Geometry check sheet. Reference: the model listing, model coordinates, mm. A direction names the side the tool comes from. Coordinates: 2 decimals unless noted, no trailing zeros. Loops run counter-clockwise (first coordinate to the right, second up) from the corner with the lowest first, then second, coordinate; pieces in that order, holes last.
Autodesk Fusion 360 part; units mm, degrees
sketch "Sketch1" plane through (0, 0, 0) normal (0, 0, 1) x (1, 0, 0)
  circle A0 centre (0, 0) radius 5.25
  circle A1 centre (0, 0) radius 6.5
  dimension "d1" = 10.5
  dimension "d2" = 1.25
sketch "Sketch2" plane through (0, 0, 0) normal (0, 0, 1) x (1, 0, 0)
  arc A0 (3.25, -8.25) -> (8.25, -3.25) centre (3.25, -3.25) ccw
  line L0 (3.25, 7.05) -> (-3.25, 7.05)
  line L1 (-8.25, 8.25) -> (8.25, -8.25) construction
  line L2 (8.25, -3.25) -> (8.25, 3.25)
  line L3 (7.05, -3.25) -> (7.05, 3.25)
  circle A1 centre (0, 0) radius 5.5
  arc A2 (-3.25, 8.25) -> (-8.25, 3.25) centre (-3.25, 3.25) ccw
  line L4 (8.25, 8.25) -> (-8.25, -8.25) construction
  line L5 (-8.25, 3.25) -> (-8.25, -3.25)
  arc A3 (-7.05, -3.25) -> (-3.25, -7.05) centre (-3.25, -3.25) ccw
  line L6 (3.25, 9.25) -> (-3.25, 9.25)
  arc A4 (-8.25, -3.25) -> (-3.25, -8.25) centre (-3.25, -3.25) ccw
  line L7 (-3.25, -7.05) -> (3.25, -7.05)
  arc A5 (8.25, 3.25) -> (3.25, 8.25) centre (3.25, 3.25) ccw
  arc A6 (3.25, -9.25) -> (9.25, -3.25) centre (3.25, -3.25) ccw
  line L8 (3.25, 8.25) -> (-3.25, 8.25)
  line L9 (9.25, -3.25) -> (9.25, 3.25)
  arc A7 (3.25, -7.05) -> (7.05, -3.25) centre (3.25, -3.25) ccw
  arc A8 (-3.25, 7.05) -> (-7.05, 3.25) centre (-3.25, 3.25) ccw
  arc A9 (-9.25, -3.25) -> (-3.25, -9.25) centre (-3.25, -3.25) ccw
  circle A10 centre (0, 0) radius 4.5
  line L10 (-3.25, -9.25) -> (3.25, -9.25)
  arc A11 (7.05, 3.25) -> (3.25, 7.05) centre (3.25, 3.25) ccw
  line L11 (-9.25, 3.25) -> (-9.25, -3.25)
  arc A12 (9.25, 3.25) -> (3.25, 9.25) centre (3.25, 3.25) ccw
  line L12 (-3.25, -8.25) -> (3.25, -8.25)
  arc A13 (-3.25, 9.25) -> (-9.25, 3.25) centre (-3.25, 3.25) ccw
  line L13 (-7.05, 3.25) -> (-7.05, -3.25)
  dimension "d3" = 1
  dimension "d4" = 1.2
  dimension "d5" = 1
  dimension "d6" = 16.5
  dimension "d7" = 16.5
  dimension "d8" = 5
  dimension "d9" = 11
extrude "Extrude1" add sketch "Sketch2" along normal blind 5 contours A0 L2 A2 L5 A4 A5 L8 L12 | A1 makes body 1 at (7.45, 1.0833, 0) makes body 2 at (5.4932, -0.2742, 3.3333)
extrude "Extrude2" add sketch "Sketch2" against normal blind 1 from surface at 5 contours A0 L2 A2 L5 A4 A5 L8 L12 | L0 L3 A3 L7 A7 A8 A11 L13 | A1 | A10 bodies 1 2
extrude "Extrude3" add sketch "Sketch1" along normal blind 13 from surface at 5 bodies 1
ref_plane "WorkPlane1" through (0, -6.5, 9.9379) normal (0, -1, 0) x (-1, 0, 0)
sketch "Sketch3" plane through (0, -6.5, 0) normal (0, -1, 0) x (-1, 0, 0)
  line L0 (0, 0) -> (0, -19) construction
  line L1 (0, 0) -> (0, -5) construction
  line L2 (0, -5) -> (0, -19) construction
  circle A0 centre (0, -12) radius 1.75
  dimension "d19" = 19
  dimension "d20" = 5
  dimension "d21" = 3.5
extrude "Extrude4" cut sketch "Sketch3" against normal blind 4 bodies 1
chamfer "Chamfer1" distance 1 angle 45 1 edges at (-6.0601, 2.3505, 5) on bodies 1
chamfer "Chamfer2" distance 1 angle 45 8 edges at (5.937, -5.937, 4) (7.05, 0, 4) (5.937, 5.937, 4) (0, 7.05, 4) (-5.937, 5.937, 4) (-7.05, 0, 4) (-5.937, -5.937, 4) (0, -7.05, 4) on bodies 1
1) Section check C-C on y = 0. Record the cut outline in (x, z).
Data:
outline: (-8.25, 0) - (-7.05, 0) - (-7.05, 3) - (-6.05, 4) - (-5.5, 4) - (-5.5, 0) - (-4.5, 0) - (-4.5, 4) - (4.5, 4) - (4.5, 0) - (5.5, 0) - (5.5, 4) - (6.05, 4) - (7.05, 3) - (7.05, 0) - (8.25, 0) - (8.25, 5) - (7.5, 5) - (6.5, 6) - (6.5, 18) - (5.25, 18) - (5.25, 5) - (-5.25, 5) - (-5.25, 18) - (-6.5, 18) - (-6.5, 6) - (-7.5, 5) - (-8.25, 5) - close
2) Section check A-A on z = 3.75. Record the cut outline in (x, y).
Data:
outline: (-8.25, -3.25) arc R5 ccw to (-3.25, -8.25) - (3.25, -8.25) arc R5 ccw to (8.25, -3.25) - (8.25, 3.25) arc R5 ccw to (3.25, 8.25) - (-3.25, 8.25) arc R5 ccw to (-8.25, 3.25) - close; circle Ø11 at (0, 0); hole (-6.3, -3.25) arc R3.05 ccw to (-3.25, -6.3) - (3.25, -6.3) arc R3.05 ccw to (6.3, -3.25) - (6.3, 3.25) arc R3.05 ccw to (3.25, 6.3) - (-3.25, 6.3) arc R3.05 ccw to (-6.3, 3.25) - close; hole circle Ø9 at (0, 0)
3) Access from +Z, -Z, +X, -X, +Y, -Y to the whole of each face (thin tool, end or side, straight path). Record for faces 5 (the flat face through (4, -7, 5)), 6 (the cylindrical face through (-5.966, 5.907, 1.479)).
Data:
face 5: +Z
face 6: -Z
4) Material ranges on probe 1 along Y at (x, z) = (0, 2.1); probe 2 along Z at (x, y) = (0, -5.4), recorded low to high.
Data:
probe 1: y = -8.25 to -7.05, -5.5 to -4.5, 4.5 to 5.5, 7.05 to 8.25
probe 2: z = 0 to 10.25, 13.75 to 18
5) Mould release check, pull along Y, two halves, no side actions. Record for faces 1 (the flat face through (0, 8.25, 2)), 2 (the cylindrical face through (-6.75, -6.82, 2.46)), 3 (the flat face through (0, -7.3, 0)), 4 (the flat face through (6.54, 0.05, 3.51)): +Y half, -Y half, draft (parallel to the pull), parting line (faces both ways), or undercut.
Data:
face 1: +Y half
face 2: -Y half
face 3: draft
face 4: undercut
6) Depth check by flat-ended pin: pin 1 (1.5 mm diameter, centred on x = -0.5, z = 15, fed in from +Y); pin 2 (3 mm diameter, centred on x = -2, y = -3, fed in from -Z); pin 3 (1 mm diameter, centred on y = -6, z = 15, fed in from +X); pin 4 (7 mm diameter, centred on x = 0, y = 0, fed in from +Z). Enter the tip coordinate at first touch or a pass-through.
Data:
pin 1: stops at y = 6.5
pin 2: stops at z = 0
pin 3: stops at x = 3.46
pin 4: stops at z = 5
7) Section check D-D on z = 1.5. Record the cut outline in (x, y), and give its area (3 significant figures).
Data:
outline: (-8.25, -3.25) arc R5 ccw to (-3.25, -8.25) - (3.25, -8.25) arc R5 ccw to (8.25, -3.25) - (8.25, 3.25) arc R5 ccw to (3.25, 8.25) - (-3.25, 8.25) arc R5 ccw to (-8.25, 3.25) - close; circle Ø11 at (0, 0); hole (-7.05, -3.25) arc R3.8 ccw to (-3.25, -7.05) - (3.25, -7.05) arc R3.8 ccw to (7.05, -3.25) - (7.05, 3.25) arc R3.8 ccw to (3.25, 7.05) - (-3.25, 7.05) arc R3.8 ccw to (-7.05, 3.25) - close; hole circle Ø9 at (0, 0)
area: 95.8 mm2
